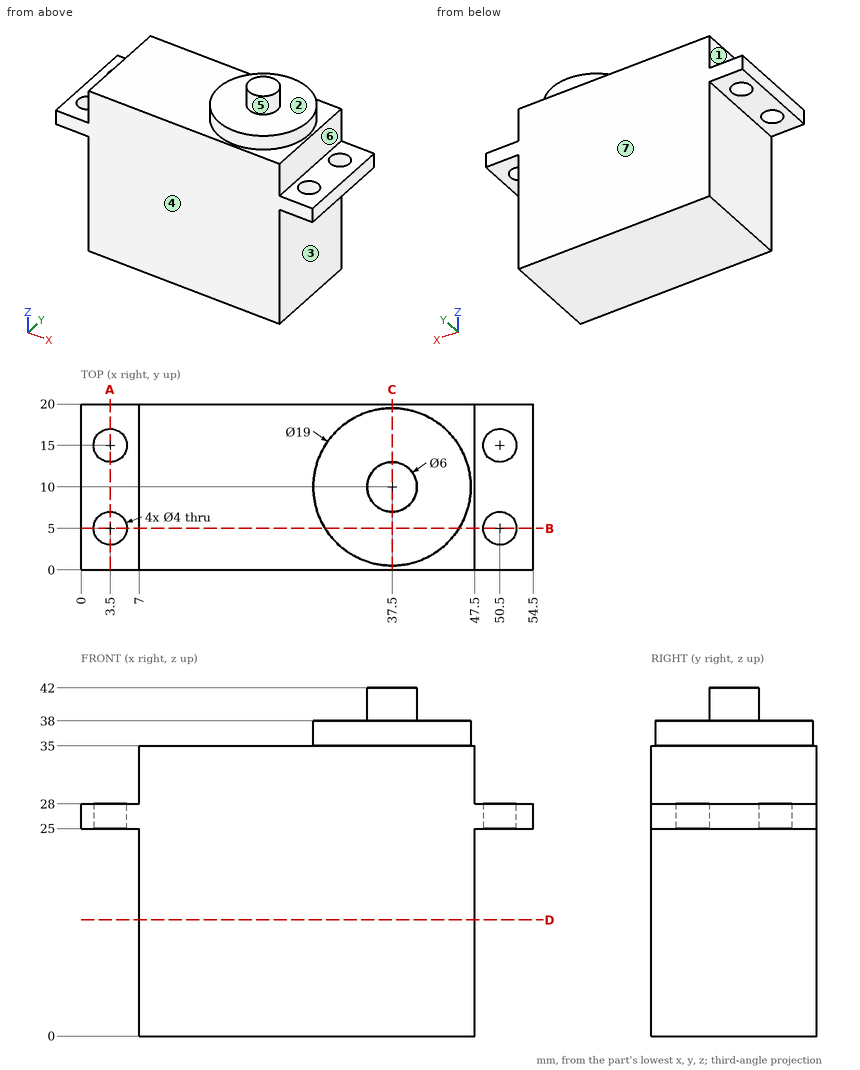
For this review, use the dimensioned drawing (mm, ordinates from the lowest corner) and the shaded views. A direction names the side the tool comes from. Coordinates: 2 decimals unless noted, no trailing zeros. Write each loop counter-clockwise with the first axis right and the second up, starting at its lowest first coordinate (ties: lowest second). Pieces come first, ordered by that corner, then holes. Notation, with made-up numbers: (-22.75, 32.5) - (-11.75, 32.5) arc R18 ccw to (-11.75, 36.5) - close; hole circle Ø6 at (-4.75, -40). An arc over 180 degrees is marked (long way). Answer in a Markdown table with one row per item. Add a question column.
Q1. Consider section D-D on z = 14. Give the boundary of the cut face in (x, y), then the cut area to 3 significant figures.
Q2. For the marked faces 1, 2 and 3, list the 3-axis set-ups (+Z, -Z, +X, -X, +Y, -Y) from which the entire face can be reached by the end or side of a thin tool; tool diameter is ignored.
Q3. To check wall thickness, follow line 1 along X through (y, z) = (5, 26.9); line 2 along Y through (x, z) = (3.5, 26.85); line 3 along Y through (x, z) = (3, 26). State the ranges of each line that lie inside material, in increasing order. Write a range as from..to.
Q4. Consider section C-C on x = 37.5. Give the boundary of the cut face in (y, z).
Q5. Consider section B-B on y = 5. Give the boundary of the cut face in (x, z).
Q6. Draft analysis for pull direction Y (two halves, no side actions). For the marked faces 4, 5, 6 and 7, state which applies: +Y half, -Y half, draft (parallel to the pull), parting line (faces both ways), or undercut.
Q7. Clearance check with flat-ended pins moving along their axes: pin 1 (1 mm diameter, centred on y = 2.5, z = 15.5, fed in from -X); pin 2 (7.5 mm diameter, centred on x = 52.5, y = 8.5, fed in from +Z); pin 3 (2 mm diameter, centred on x = 3.5, y = 12, fed in from -Z). State where each tip first meets the part, or that it passes through.
Q8. Consider section A-A on x = 3.5. Give the boundary of the cut face in (y, z).
Answers below:
| question | item | result |
|---|---|---|
| 1 | outline | (7, 0) - (47.5, 0) - (47.5, 20) - (7, 20) - close |
| 1 | area | 810 mm² |
| 2 | face 1 | +Z, -X, +Y, -Y |
| 2 | face 2 | +Z |
| 2 | face 3 | -Z, +X, +Y, -Y |
| 3 | line 1 | 0..1.5, 5.5..48.5, 52.5..54.5 |
| 3 | line 2 | 0..3, 7..13, 17..20 |
| 3 | line 3 | 0..3.06, 6.94..13.06, 16.94..20 |
| 4 | outline | (0, 0) - (20, 0) - (20, 35) - (19.5, 35) - (19.5, 38) - (13, 38) - (13, 42) - (7, 42) - (7, 38) - (0.5, 38) - (0.5, 35) - (0, 35) - close |
| 5 | outline | (0, 25) - (1.5, 25) - (1.5, 28) - (0, 28) - close; (5.5, 25) - (7, 25) - (7, 0) - (47.5, 0) - (47.5, 25) - (48.5, 25) - (48.5, 28) - (47.5, 28) - (47.5, 35) - (45.58, 35) - (45.58, 38) - (29.42, 38) - (29.42, 35) - (7, 35) - (7, 28) - (5.5, 28) - close; (52.5, 25) - (54.5, 25) - (54.5, 28) - (52.5, 28) - close |
| 6 | face 4 | -Y half |
| 6 | face 5 | parting line |
| 6 | face 6 | draft |
| 6 | face 7 | +Y half |
| 7 | pin 1 | x = 7 |
| 7 | pin 2 | z = 28 |
| 7 | pin 3 | z = 25 |
| 8 | outline | (0, 25) - (3, 25) - (3, 28) - (0, 28) - close; (7, 25) - (13, 25) - (13, 28) - (7, 28) - close; (17, 25) - (20, 25) - (20, 28) - (17, 28) - close |
